from build123d import *

# Parameters (mm, degrees)
F0_R     = 2.667
F0_R_2   = 2.625
F2_DEPTH = 6
F3_DEPTH = 3.5
F4_DEPTH = 4
F5_DEPTH = 10
F1_R     = 1
F6_DEPTH = 18.001
F7_R     = 4.99999


# Not quite as in the source:
# - a fillet or chamfer is up to 0.001 mm smaller than in the source, because OpenCascade refuses the exact size


with BuildPart() as f2:
    # F0 (on Right) → F2 (new body)
    with BuildSketch(Plane.YZ):
        Polygon((7.0520542562, 18), (-12.9479457438, 18), (-12.9479457438, 10), (-2.9479457438, 10), (7.0520542562, 10), align=None)
        with BuildLine():
            Line((22.0520542562, 18), (7.0520542562, 18))
            Line((7.0520542562, 18), (7.0520542562, 10))
            Line((7.0520542562, 10), (17.0520542562, 10))
            Line((17.0520542562, 10), (27.0520542562, 10))
            Line((27.0520542562, 10), (27.0520542562, 13))
            ThreePointArc((27.0520542562, 13), (25.5875881621, 16.5355339059), (22.0520542562, 18))
        make_face()
        with BuildLine():
            Line((-2.9479457438, 10), (-12.9479457438, 10))
            Line((-12.9479457438, 10), (-12.9479457438, 0))
            ThreePointArc((-12.9479457438, 0), (-11.4834796497, -3.5355339059), (-7.9479457438, -5))
            ThreePointArc((-7.9479457438, -5), (-4.4124118379, -3.5355339059), (-2.9479457438, 0))
            Line((-2.9479457438, 0), (-2.9479457438, 10))
        make_face()
        with Locations((-7.9479457438, 0)):
            Circle(F0_R, mode=Mode.SUBTRACT)
        with BuildLine():
            Line((27.0520542562, 10), (17.0520542562, 10))
            Line((17.0520542562, 10), (17.0520542562, 0))
            ThreePointArc((17.0520542562, 0), (18.5165203503, -3.5355339059), (22.0520542562, -5))
            ThreePointArc((22.0520542562, -5), (25.5875881621, -3.5355339059), (27.0520542562, 0))
            Line((27.0520542562, 0), (27.0520542562, 10))
        make_face()
        with Locations((22.0520542562, 0)):
            Circle(F0_R_2, mode=Mode.SUBTRACT)
        with Locations((-7.9479457438, 0)):
            Circle(F0_R)
        with Locations((22.0520542562, 0)):
            Circle(F0_R_2)
    extrude(amount=-F2_DEPTH)

    # F0 (on Right) → F3 (join)
    with BuildSketch(Plane.YZ):
        with Locations((22.0520542562, 0)):
            Circle(F0_R_2)
    extrude(amount=F3_DEPTH)

    # F0 (on Right) → F4 (cut)
    with BuildSketch(Plane.YZ):
        with Locations((-7.9479457438, 0)):
            Circle(F0_R)
    extrude(amount=-F4_DEPTH, mode=Mode.SUBTRACT)

    # F0 (on Right) → F5 (join)
    with BuildSketch(Plane.YZ):
        Polygon((7.0520542562, 18), (-12.9479457438, 18), (-12.9479457438, 10), (-2.9479457438, 10), (7.0520542562, 10), align=None)
    extrude(amount=F5_DEPTH)

    # F1 (on Top) → F6 (cut, through all)
    with BuildSketch(Plane.XY):
        with Locations((2.75, 1.5520542562)):
            Circle(F1_R)
        with Locations((2.75, -7.9479457438)):
            Circle(F1_R)
    extrude(amount=F6_DEPTH, mode=Mode.SUBTRACT)

    # F7 (radius 5 in the source; OpenCascade refuses exactly that, so slightly less here)
    f7_edges = [f2.edges().sort_by_distance(p)[0] for p in [
        (0, 7.052054, 14),
        (-3, -2.947946, 10),
        (-3, 17.052054, 10),
    ]]
    fillet(f7_edges, radius=F7_R)


solid = f2.part
The listing builds one solid part. Answer for the finished solid, in the listing's coordinates (mm). A direction names the side the tool comes from. Coordinates: 2 decimals unless noted, no trailing zeros. Write each loop counter-clockwise with the first axis right and the second up, starting at its lowest first coordinate (ties: lowest second). Pieces come first, ordered by that corner, then holes. Notation, with made-up numbers: (65, 70) - (96, 70) arc R25 ccw to (96, 84) - close; hole circle Ø3 at (37.5, 53.5). An arc over 180 degrees is marked (long way). Answer as CSV lines item,"result".
1. Find section B-B (x = 2.75). Give the vertices of the cut face in (y, z) (3 decimals).
Computed values:
outline,"(-12.948, 10) - (-8.948, 10) - (-8.948, 18) - (-12.948, 18) - close; (-6.948, 10) - (0.552, 10) - (0.552, 18) - (-6.948, 18) - close; (2.552, 10) - (7.587, 10) - (7.587, 18) - (2.552, 18) - close; circle Ø5.25 at (22.052, 0)"
2. Given P1, Ø7.5, axis at y = -8.5, z = 3.5, coming from the +X side; P2, Ø5, axis at x = -1.5, y = 3.5, coming from the -Z side; P3, Ø4, axis at y = 22, z = -0.5, coming from the +X side; P4, Ø2.5, axis at x = 2.75, y = 1.55, coming from the +Z side, each flat-ended and moving along its own axis, determine where each tip first touches the part or whether it passes through.
Computed values:
P1,"stops at x = 0"
P2,"stops at z = 9.89"
P3,"stops at x = 3.5"
P4,"stops at z = 18"
3. Straight lines are drawn through the part: line 1 (Y direction, x = 2.75, z = 12.75); line 2 (X direction, y = 24.5, z = 13.25); line 3 (Z direction, x = -2.5, y = -10). For each, find the intervals that lie inside material, in ascending order. Write a range as [from, to].
Computed values:
line 1,"y = [-12.95, -8.95], [-6.95, 0.55], [2.55, 7.59]"
line 2,"x = [-6, 0]"
line 3,"z = [-4.56, -1.7], [1.7, 18]"
4. Find section C-C (z = 14.75). Give the vertices of the cut face in (x, y), plus the area to 3 significant figures.
Computed values:
outline,"(-6, -12.95) - (10, -12.95) - (10, 7.05) - (5, 7.05) arc R5 cw to (0, 12.05) - (0, 26.74) - (-6, 26.74) - close; hole circle Ø2 at (2.75, -7.95); hole circle Ø2 at (2.75, 1.55)"
area,"437 mm²"
5. A tool of negligible diameter and unlimited length cuts with its end or side. For faces 5 (the flat face through (0, -7, 4)), 6 (the flat face through (7, 7.052, 14)), 7 (the cylindrical face through (-3.04, 15.55, 8.57)), 8 (the flat face through (2, -1, 10)), 9 (the cylindrical face through (1.726, 24.477, -1.005)), from which of +Z, -Z, +X, -X, +Y, -Y can it reach the whole face along a straight path? Write none if from no direction.
Computed values:
face 5,"-Z, +X, -Y"
face 6,"+Z, -Z, +X, +Y"
face 7,"-Z, +X, -X"
face 8,"-Z, +X"
face 9,"+X"
6. Determine the mould class of faces 1 (the cylindrical face through (-1.972, -10.612, 0.117)), 2 (the cylindrical face through (-3.042, -1.444, 8.574)), 3 (the flat face through (-4, -8, 0)), 4 (the cylindrical face through (1.75, 1.6, 13.94)) for opening direction Z: +Z half, -Z half, draft (parallel to the pull), parting line (faces both ways), or undercut.
Computed values:
face 1,"undercut"
face 2,"-Z half"
face 3,"undercut"
face 4,"draft"
7. Find section A-A (z = 4). Give the vertices of the cut face in (x, y), plus the area to 3 significant figures.
Computed values:
outline,"(-6, -12.95) - (0, -12.95) - (0, -2.95) - (-6, -2.95) - close; (-6, 17.05) - (0, 17.05) - (0, 27.05) - (-6, 27.05) - close"
area,"120 mm²"
8. Find section D-D (z = -0.75). Give the vertices of the cut face in (x, y), plus the area to 3 significant figures.
Computed values:
outline,"(-6, -12.89) - (0, -12.89) - (0, -10.51) - (-4, -10.51) - (-4, -5.39) - (0, -5.39) - (0, -3) - (-6, -3) - close; (-6, 17.11) - (0, 17.11) - (0, 19.54) - (3.5, 19.54) - (3.5, 24.57) - (0, 24.57) - (0, 27) - (-6, 27) - close"
area,"116 mm²"
